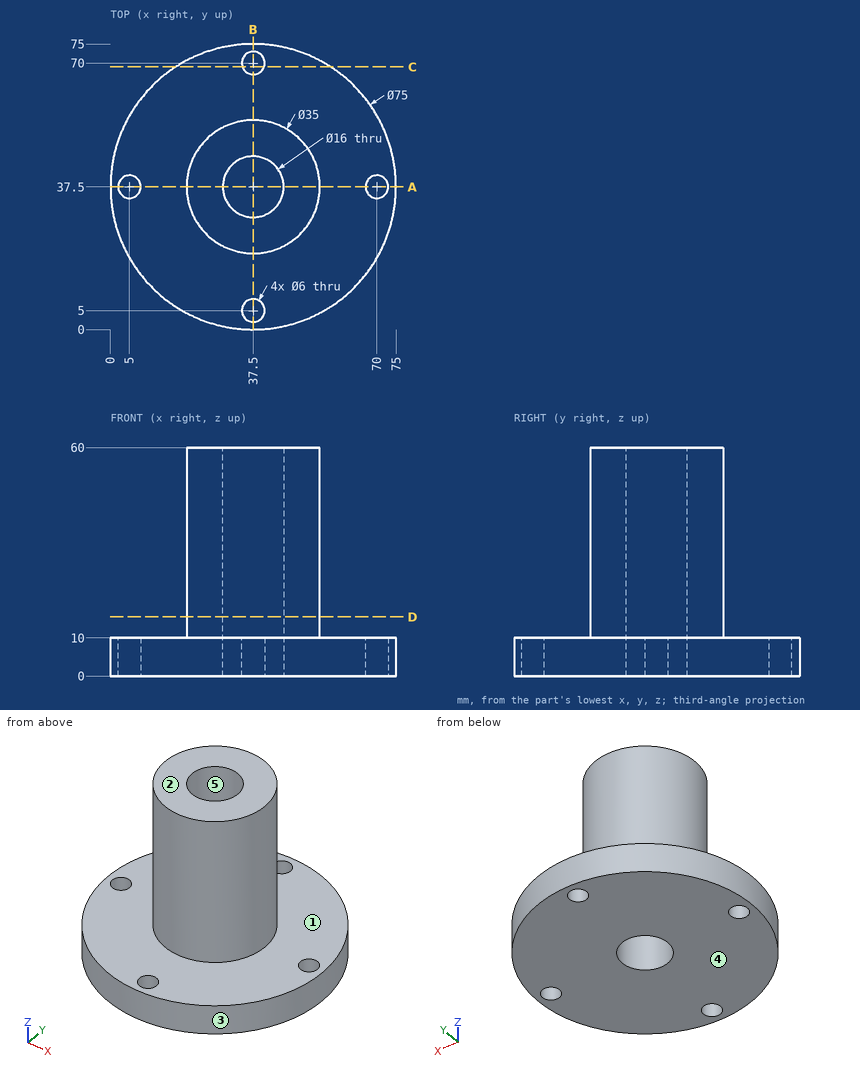
Job drawing, mm, ordinate dimensions from the low corner. One solid piece. A direction names the side the tool comes from. Give positions to 0.01 mm unless a question says otherwise; leave off trailing zeros. Order: outer loops, then holes, each group sorted by start corner. A loop starts at its lowest first (then second) coordinate and runs counter-clockwise, first axis right, second up. Notation, with made-up numbers: (73, 88.5) - (101, 88.5) arc R20 cw to (101, 120.5) - close; hole circle Ø4 at (38.25, 37.25). An arc over 180 degrees is marked (long way). Return JSON: item names as keys, results as strings.
1) Cut at D-D, the plane z = 15.5. Give the cut face in (x, y), plus the area to 3 significant figures.
Geometry says:
{"outline": "circle Ø35 at (37.5, 37.5); hole circle Ø16 at (37.5, 37.5)", "area": "761 mm²"}
2) Flat gauge pins, fed straight in: P1, Ø1.5, axis at y = 51.5, z = 7, coming from the -X side; P2, Ø8, axis at x = 37.5, y = 70, coming from the +Z side; P3, Ø12, axis at y = 16.5, z = 39, coming from the -X side; P4, Ø6, axis at x = 24, y = 24.5, coming from the +Z side. Where does each tip first touch, or does it go through?
Geometry says:
{"P1": "x = 2.42", "P2": "z = 10", "P3": "x = 28.49", "P4": "z = 60"}
3) Probe line 1 (Y direction, x = 36.5, z = 9); line 2 (X direction, y = 37, z = 40). List the from-to ranges inside material, lowest first. Write a range as from..to.
Geometry says:
{"line 1": "0.01..2.17, 7.83..29.56, 45.44..67.17, 72.83..74.99", "line 2": "20.01..29.52, 45.48..54.99"}
4) Pull direction X, two halves, no side cores. Call the marked faces 3, 4 and 5: pulls with the +X half, pulls with the -X half, needs draft (parallel to the pull), parting line crosses it, or undercut.
Geometry says:
{"face 3": "parting line crosses it", "face 4": "needs draft", "face 5": "undercut"}
5) Cut at C-C, the plane y = 69. Give the cut face in (x, z).
Geometry says:
{"outline": "(17.15, 0) - (34.67, 0) - (34.67, 10) - (17.15, 10) - close; (40.33, 0) - (57.85, 0) - (57.85, 10) - (40.33, 10) - close"}
6) 3-axis set-ups, long thin cutter, end or side, ignore diameter. For the marked faces 1 and 2: which of +Z, -Z, +X, -X, +Y, -Y reach the whole face in a straight line?
Geometry says:
{"face 1": "+Z", "face 2": "+Z, +X, -X, +Y, -Y"}
7) Cut at A-A, the plane y = 37.5. Give the cut face in (x, z).
Geometry says:
{"outline": "(0, 0) - (2, 0) - (2, 10) - (0, 10) - close; (8, 0) - (29.5, 0) - (29.5, 60) - (20, 60) - (20, 10) - (8, 10) - close; (45.5, 0) - (67, 0) - (67, 10) - (55, 10) - (55, 60) - (45.5, 60) - close; (73, 0) - (75, 0) - (75, 10) - (73, 10) - close"}
